Autodesk Inventor part; units mm, degrees
ref_plane "YZ Plane" through (0, 0, 0) normal (1, 0, 0) x (0, 1, 0)
ref_plane "XZ Plane" through (0, 0, 0) normal (0, 1, 0) x (-1, 0, 0)
ref_plane "XY Plane" through (0, 0, 0) normal (0, 0, 1) x (1, 0, 0)
sketch "Sketch2" plane through (0, 0, 0) normal (0, 0, 1) x (1, 0, 0)
  line L0 (-14.5, 10) -> (14.5, 10)
  line L1 (14.5, 10) -> (14.5, 27.5)
  line L2 (14.5, 27.5) -> (12.5, 27.5)
  line L3 (12.5, 27.5) -> (12.5, 23)
  line L4 (12.5, 23) -> (-12.5, 23)
  line L5 (-12.5, 23) -> (-12.5, 27.5)
  line L6 (-12.5, 27.5) -> (-14.5, 27.5)
  line L7 (-14.5, 27.5) -> (-14.5, 10)
  line L8 (0, 0) -> (-7.6194, 0) construction
  line L9 (0, 0) -> (0, 10) construction
  dimension "d11" = 20
  dimension "d12" = 55
  dimension "d13" = 2
  dimension "d14" = 29
  dimension "d15" = 46
revolve "Revolution1" add sketch "Sketch2" angle 360 about axis through (0, 0, 0) along (-1, 0, 0)
properties part number "Solder Spool" material "SAE 1020"
Build history of the part. All positions in model axes, mm. A direction names the side the tool comes from. Coordinates: 2 decimals unless noted, no trailing zeros. Order: outer loops, then holes, each group sorted by start corner. A loop starts at its lowest first (then second) coordinate and runs counter-clockwise, first axis right, second up. Notation, with made-up numbers: (-22, 53) -> (-2, 53) arc R16 ccw to (-2, 57) -> close; hole circle Ø2 at (25.25, 74). An arc over 180 degrees is marked (long way). Answer in a Markdown table with one row per item. Add a question column.
Q1. Band-saw the part on A-A, the plane y = 0. List the corners of the cut face in (x, z), then the cut area to 3 significant figures.
Q2. Mould opens along Z. For faces 1 (the face through (0.2, -2.17, -9.76)), 2 (the face through (-13.514, -5.961, 26.846)), 3 (the face through (-14.5, 0, 12)) say: +Z half, -Z half, draft (parallel to the pull), parting line (faces both ways), or undercut.
Q3. Band-saw the part on D-D, the plane z = -19.5. List the corners of the cut face in (x, y).
Q4. Which spindle directions (+Z, -Z, +X, -X, +Y, -Y) get a long thin tool onto all of the face, cutting with end or side? Do faces 4 (the face through (-12.5, -14.4, 18.2)), 5 (the face through (14.5, 0, 12)). Say none if no direction does.
Q5. Drop flat-ended pins along their axis: pin 1 (3 mm diameter, centred on x = -6.5, y = -18.5, fed in from -Z); pin 2 (10 mm diameter, centred on x = 4, z = 4, fed in from -Y); pin 3 (1 mm diameter, centred on x = 2.5, y = 0.5, fed in from +Z); pin 4 (12 mm diameter, centred on y = 0, z = 0, fed in from -X). Give the stop position or say it passes through.
Q6. Band-saw the part on C-C, the plane x = -5.75. List the corners of the cut face in (y, z).
Q7. Wall check: line 1 along X through (y, z) = (1, -23.5); line 2 along Z through (x, y) = (6, 0); line 3 along Y through (x, z) = (-11.75, -0.5). Give the ranges that are in metal, low to high. Write a range as [from, to].
Q8. Band-saw the part on B-B, the plane z = -9. List the corners of the cut face in (x, y).
Answers follow:
| question | item | result |
|---|---|---|
| 1 | outline | (-14.5, -27.5) -> (-12.5, -27.5) -> (-12.5, -23) -> (12.5, -23) -> (12.5, -27.5) -> (14.5, -27.5) -> (14.5, -10) -> (-14.5, -10) -> close; (-14.5, 10) -> (14.5, 10) -> (14.5, 27.5) -> (12.5, 27.5) -> (12.5, 23) -> (-12.5, 23) -> (-12.5, 27.5) -> (-14.5, 27.5) -> close |
| 1 | area | 790 mm^2 |
| 2 | face 1 | undercut |
| 2 | face 2 | parting line |
| 2 | face 3 | draft |
| 3 | outline | (-14.5, -19.39) -> (-12.5, -19.39) -> (-12.5, -12.2) -> (12.5, -12.2) -> (12.5, -19.39) -> (14.5, -19.39) -> (14.5, 19.39) -> (12.5, 19.39) -> (12.5, 12.2) -> (-12.5, 12.2) -> (-12.5, 19.39) -> (-14.5, 19.39) -> close |
| 4 | face 4 | none |
| 4 | face 5 | +Z, -Z, +X, +Y, -Y |
| 5 | pin 1 | z = -15.49 |
| 5 | pin 2 | y = -23 |
| 5 | pin 3 | z = 23 |
| 5 | pin 4 | through |
| 6 | outline | circle Ø46 at (0, 0); hole circle Ø20 at (0, 0) |
| 7 | line 1 | [-14.5, -12.5], [12.5, 14.5] |
| 7 | line 2 | [-23, -10], [10, 23] |
| 7 | line 3 | [-22.99, -9.99], [9.99, 22.99] |
| 8 | outline | (-14.5, -25.99) -> (-12.5, -25.99) -> (-12.5, -21.17) -> (12.5, -21.17) -> (12.5, -25.99) -> (14.5, -25.99) -> (14.5, -4.36) -> (-14.5, -4.36) -> close; (-14.5, 4.36) -> (14.5, 4.36) -> (14.5, 25.99) -> (12.5, 25.99) -> (12.5, 21.17) -> (-12.5, 21.17) -> (-12.5, 25.99) -> (-14.5, 25.99) -> close |
